Work out the finished part from the listing and answer in its coordinate system (mm). A direction names the side the tool comes from. Coordinates: 2 decimals unless noted, no trailing zeros. Order: outer loops, then holes, each group sorted by start corner. A loop starts at its lowest first (then second) coordinate and runs counter-clockwise, first axis right, second up.
1. Flat-ended cylindrical pins translate along their axes: pin 1 Ø8 at (y, z) = (-5, -1.5) entering from -X; pin 2 Ø2 at (x, y) = (2, 9) entering from -Z; pin 3 Ø4 at (x, y) = (5, 7.5) entering from +Z; pin 4 Ø6 at (x, y) = (-10, -2.5) entering from -Z. Find the tip coordinate at first contact, or state that the pin passes through.
2. The part is cut by section D-D, the plane y = -2. Give the vertices of the cut face in (x, z), then the cut area to 3 significant figures.
3. Find the intervals of material crossed by probe 1 along Z at (x, y) = (0, 10.5); probe 2 along Z at (x, y) = (-4, 6.25); probe 3 along X at (y, z) = (10.25, -2), in increasing order.
4. A tool of negligible diameter and unlimited length cuts with its end or side. For faces 1 (the cylindrical face through (-0.59, -0.16, 4.46)), 2 (the cylindrical face through (0.75, 14.7, -0.03)), 3 (the flat face through (0, -11.673, 0)), from which of +Z, -Z, +X, -X, +Y, -Y can it reach the whole face along a straight path? Write none if from no direction.
5. The part is cut by section C-C, the plane y = 15.25. Give the vertices of the cut face in (x, z), then the cut area to 3 significant figures.
Solid Edge part; units mm, degrees
sketch "Sketch1" plane through (0, 0, 0) normal (0, -1, 0) x (1, 0, 0)
  circle A0 centre (0, 0) radius 4.5
extrude "Protrusion1" add sketch "Sketch1" along normal mid plane 23.3462
sketch "Sketch2" plane through (0, 11.6731, 0) normal (0, 1, 0) x (-1, 0, 0)
  circle A0 centre (0, 0) radius 0.75
extrude "ExtrudedProtrusion_2" add sketch "Sketch2" along normal mid plane 12.2854
sketch "Sketch3" plane through (0, 17.8158, 0) normal (0, 1, 0) x (-1, 0, 0)
  circle A0 centre (0, 0) radius 15.3384
extrude "ExtrudedProtrusion_3" add sketch "Sketch3" along normal mid plane 0.01
Geometry says:
1. pin 1: stops at x = -4.5
1. pin 2: stops at z = -4.39
1. pin 3: stops at z = 3.35
1. pin 4: passes through
2. outline: circle Ø9 at (0, 0)
2. area: 63.6 mm2
3. probe 1: z = -4.5 to 4.5
3. probe 2: z = -2.06 to 2.06
3. probe 3: x = -4.03 to 4.03
4. face 1: -Y
4. face 2: none
4. face 3: +Z, -Z, +X, -X, -Y
5. outline: circle Ø1.5 at (0, 0)
5. area: 1.77 mm2
